Can you work these out from the model? Positions are in its coordinate system, mm. Coordinates: 2 decimals unless noted, no trailing zeros. Order: outer loops, then holes, each group sorted by start corner. A loop starts at its lowest first (then second) coordinate and runs counter-clockwise, first axis right, second up. Notation, with made-up numbers: (59, 69) -> (87, 69) arc R9 ccw to (87, 81) -> close; hole circle Ø11 at (50.5, 46). An arc over 180 degrees is marked (long way). Answer in a Markdown table with one row per item.
Autodesk Inventor part; units mm, degrees
ref_plane "YZ Plane" through (0, 0, 0) normal (1, 0, 0) x (0, 1, 0)
ref_plane "XZ Plane" through (0, 0, 0) normal (0, 1, 0) x (-1, 0, 0)
ref_plane "XY Plane" through (0, 0, 0) normal (0, 0, 1) x (1, 0, 0)
sketch "Sketch1" plane through (0, 0, 0) normal (1, 0, 0) x (0, 1, 0)
  line L0 (0, 100) -> (-100, 100)
  line L1 (-100, 100) -> (-100, -100)
  line L2 (-100, -100) -> (100, -100)
  line L3 (100, -100) -> (100, 100)
  line L4 (100, 100) -> (0, 100)
  point P0 (0, 0)
  dimension "d1" = 100
  dimension "d2" = 200
  dimension "d3" = 200
  dimension "d4" = 200
extrude "Extrusion1" add sketch "Sketch1" along normal blind 20
sketch "Sketch2" plane through (0, 0, 0) normal (-1, 0, 0) x (0, 0, 1)
  circle A0 centre (-56.5685, 56.5685) radius 4
  point P0 (0, 0)
  dimension "d11" = 8
extrude "Extrusion2" cut sketch "Sketch2" against normal blind 20
pattern_circular "Circular Pattern1" count 4 over 360 about axis through (-10, 0, 0) along (1, 0, 0) of "Extrusion2"
sketch "Sketch3" plane through (0, 0, 0) normal (-1, 0, 0) x (0, 0, 1)
  circle A0 centre (-56.5685, -56.5685) radius 4
  circle A1 centre (56.5685, -56.5685) radius 4
  circle A2 centre (0, -56.5685) radius 4
  point P0 (0, 0)
  dimension "d17" = 8
extrude "Extrusion3" cut sketch "Sketch3" against normal blind 20 contours A2
properties part number "TMP_fix_plate"
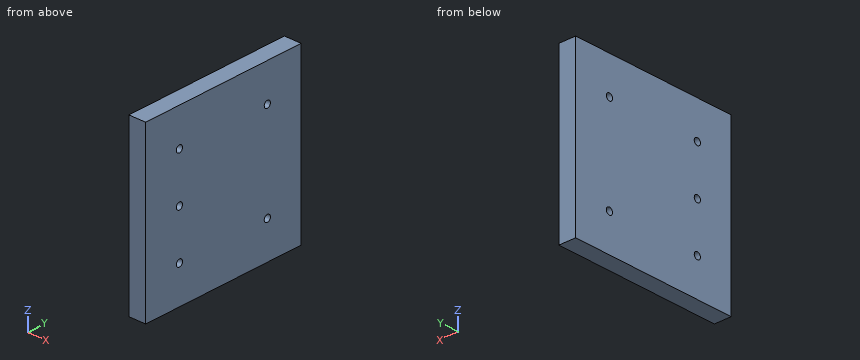
(1) Will this pin go through, and if not, where does the flat tip stop? pin 1 Ø10.5 at (y, z) = (-56.57, 0) entering from +X.
Response values:
| item | result |
|---|---|
| pin 1 | x = 20 |
(2) I need wall thicknesses on line 1 (Y direction, x = 2.25, z = 58); line 2 (Y direction, x = 1.25, z = 55); line 3 (Z direction, x = 17.75, y = -60). Which ranges of each line are inside material? Lowest first, please. Write a range as [from, to].
Response values:
| item | result |
|---|---|
| line 1 | [-100, -60.3], [-52.83, 52.83], [60.3, 100] |
| line 2 | [-100, -60.25], [-52.89, 52.89], [60.25, 100] |
| line 3 | [-100, -58.62], [-54.51, -2.06], [2.06, 54.51], [58.62, 100] |
(3) Suppose I cut it at A-A (z = 0). Please give me the cut outline in (x, y).
Response values:
| item | result |
|---|---|
| outline | (0, -100) -> (20, -100) -> (20, -60.57) -> (0, -60.57) -> close; (0, -52.57) -> (20, -52.57) -> (20, 100) -> (0, 100) -> close |
